For this review, take the finished solid that the model builds, in its own axes (mm). A direction names the side the tool comes from. Give positions to 0.01 mm unless a question says otherwise; leave off trailing zeros. Write each loop counter-clockwise with the first axis right and the second up, starting at its lowest first coordinate (ties: lowest second). Pieces come first, ordered by that corner, then holes. Notation, with made-up numbers: M -31.5,5 L -27.5,5 A13 ccw -27.5,16 Z; hole C 85,1.25 d8. An arc over 180 degrees is marked long. Use one line per item in the form item = value. Start each with the question number.
Q1. Consider section B-B on y = 6. Write out the cut boundary in (x, z).
Q2. Consider section C-C on z = 12.5. Give the number of separate pieces and of enclosed holes in the cut face, and give its area (3 significant figures).
Q3. For probe 1 along Z at (x, y) = (-30, -39); probe 2 along Z at (x, y) = (-30, -32.5); probe 3 along Y at (x, z) = (-7.75, 2.05), list the stretches that pass through material, from the lowest coordinate up. Write a range as [from, to].
Q4. Consider section A-A on x = 0. Write out the cut boundary in (y, z), and give its area (3 significant figures).
Q5. Consider section D-D on x = 12. Write out the cut boundary in (y, z).
Q6. Mouldability with a two-part tool opening along Y and no side actions: class faces 1 (the flat face through (8, 0, 3)), 2 (the flat face through (-40, -42, 12)), 3 (the flat face through (0, -38, 13)) as released by +Y, released by -Y, zero draft, split by the parting line, or undercut.
Q7. Clearance check with flat-ended pins moving along their axes: pin 1 Ø5 at (x, y) = (-7.75, 13.42) entering from +Z; pin 2 Ø6 at (x, z) = (33, 10.5) entering from +Y; pin 3 Ø8 at (y, z) = (-28.5, 17) entering from +X; pin 4 Ø2.5 at (x, y) = (15.5, 0) entering from -Z. State where each tip first meets the part, or that it passes through.
Q8. Tool access review of faces 4 (the flat face through (27, -35, 10)), 5 (the cylindrical face through (-1.517, -41.549, 5.666)), 6 (the flat face through (20.5, -8, 12)), 7 (the cylindrical face through (-23.416, -26.115, 12.675)), 8 (the cylindrical face through (0.1, -13.1, 1.5)): name each direction out of +Z, -Z, +X, -X, +Y, -Y from which nothing blocks a thin tool from reaching the whole face with its end or side.
Autodesk Fusion 360 part; units mm, degrees
sketch "Sketch1" plane through (0, 0, 0) normal (0, 0, 1) x (1, 0, 0)
  circle A0 centre (0, 0) radius 15.5 construction
  circle A1 centre (0, 0) radius 18.5
  circle A2 centre (0, 0) radius 20.5
  line L0 (-18.5, 0) -> (18.5, 0) construction
  circle A3 centre (-15.5, 0) radius 1.6
  circle A4 centre (15.5, 0) radius 1.6
  circle A5 centre (7.75, -13.4234) radius 1.6
  circle A6 centre (-7.75, -13.4234) radius 1.6
  circle A7 centre (7.75, 13.4234) radius 1.6
  circle A8 centre (-7.75, 13.4234) radius 1.6
  line L1 (0, 18.5) -> (0, -40) construction
  line L2 (40, -45) -> (-40, -45)
  line L3 (-40, -45) -> (-40, -35)
  line L4 (-40, -35) -> (40, -35)
  line L5 (40, -35) -> (40, -45)
  line L6 (40, -45) -> (-40, -35) construction
  line L7 (-40, -45) -> (40, -35) construction
  line L8 (-20.5, -35) -> (-20.5, 0)
  line L9 (20.5, -35) -> (20.5, 0)
  circle A9 centre (0, 7) radius 6.1
  circle A10 centre (0, -7) radius 6.1
  line L10 (-6.1, -7) -> (-6.1, 7)
  line L11 (6.1, 7) -> (6.1, -7)
  dimension "d1" = 31
  dimension "d2" = 37
  dimension "d3" = 2
  dimension "d4" = 3.2
  dimension "d5" = 3.2
  dimension "d6" = 3.2
  dimension "d7" = 3.2
  dimension "d8" = 3.2
  dimension "d9" = 3.2
  dimension "d10" = 15.5
  dimension "d11" = 15.5
  dimension "d12" = 15.5
  dimension "d13" = 15.5
  dimension "d14" = 15.5
  dimension "d21" = 10
  dimension "d22" = 80
  dimension "d32" = 12.2
  dimension "d33" = 7
  dimension "d52" = 35
extrude "Extrude1" add sketch "Sketch1" along normal blind 3 contours A1
extrude "Extrude2" add sketch "Sketch1" along normal blind 25 contours A2 | A2 L4 L8 L9 | L2 L3 L4 L5
sketch "Sketch6" plane through (0, -35, 0) normal (0, 1, 0) x (-1, 0, 0)
  line L0 (20.5, 0) -> (40, 0)
  line L1 (40, 0) -> (40, 25)
  line L2 (40, 25) -> (20.5, 25)
  line L3 (20.5, 25) -> (20.5, 0)
  line L4 (-40, 0) -> (-20.5, 0)
  line L5 (-20.5, 0) -> (-20.5, 25)
  line L6 (-20.5, 25) -> (-40, 25)
  line L7 (-40, 25) -> (-40, 0)
  line L8 (-40, 12.5) -> (40, 12.5) construction
  circle A0 centre (-30, 12.5) radius 3.1
  line L9 (0, 0) -> (0, 42.7428) construction
  circle A1 centre (30, 12.5) radius 3.1
  circle A2 centre (30, 12.5) radius 6
  circle A3 centre (-30, 12.5) radius 6
  dimension "d42" = 6.2
  dimension "d43" = 6.2
  dimension "d44" = 30
  dimension "d45" = 30
  dimension "d46" = 12
  dimension "d47" = 12
fillet "Fillet2" radius 19 2 edges at (20.5, -35, 12.5) (-20.5, -35, 12.5)
extrude "Extrude3" cut sketch "Sketch6" against normal through all contours A0 | A1
extrude "Extrude4" cut sketch "Sketch6" along normal through all contours A0 | A1 | A2 | A3
fillet "Fillet3" radius 4 2 edges at (40, -35, 12.5) (-40, -35, 12.5)
sketch "Sketch7" plane through (0, -45, 0) normal (0, -1, 0) x (1, 0, 0)
  circle A0 centre (30, 12.5) radius 3.1
  circle A1 centre (-30, 12.5) radius 3.1
  line L0 (-40, 0) -> (40, 0)
  line L1 (40, 0) -> (40, 25)
  line L2 (40, 25) -> (-40, 25)
  line L3 (-40, 25) -> (-40, 0)
  line L4 (-30, 12.5) -> (30, 12.5) construction
  circle A2 centre (0, 12.5) radius 7
  dimension "d55" = 14
extrude "Extrude7" cut sketch "Sketch7" against normal blind 7 contours A2
Working result:
q1.outline = M -19.6,0 L -6.1,0 L -6.1,3 L -17.5,3 L -17.5,25 L -19.6,25 Z; M 6.1,0 L 19.6,0 L 19.6,25 L 17.5,25 L 17.5,3 L 6.1,3 Z
q2.separate_pieces = 3
q2.enclosed_holes = 1
q2.area = 1,670 mm²
q3.probe_1 = [0, 9.4], [15.6, 25]
q3.probe_2 = [0, 6.5], [18.5, 25]
q3.probe_3 = [-45, -15.02], [-11.82, 11.82], [15.02, 18.98]
q4.outline = M -45,0 L -13.1,0 L -13.1,3 L -18.5,3 L -18.5,25 L -45,25 L -45,19.5 L -38,19.5 L -38,5.5 L -45,5.5 Z; M 13.1,0 L 20.5,0 L 20.5,25 L 18.5,25 L 18.5,3 L 13.1,3 Z
q4.area = 647 mm²
q5.outline = M -45,0 L 16.62,0 L 16.62,25 L 14.08,25 L 14.08,3 L -14.08,3 L -14.08,25 L -45,25 Z
q6.face_1 = undercut
q6.face_2 = zero draft
q6.face_3 = released by -Y
q7.pin_1 = 3
q7.pin_2 = -33.98
q7.pin_3 = 29.59
q7.pin_4 = through
q8.face_4 = +Y
q8.face_5 = -Y
q8.face_6 = +Z, -Z, +X, +Y
q8.face_7 = +Z, -Z, -X, +Y
q8.face_8 = +Z, -Z
